Here's how the part is built. I have some questions about the finished solid (model axes, mm). A direction names the side the tool comes from. Coordinates: 2 decimals unless noted, no trailing zeros. Order: outer loops, then holes, each group sorted by start corner. A loop starts at its lowest first (then second) coordinate and runs counter-clockwise, first axis right, second up. Notation, with made-up numbers: (5, 8.25) - (31, 8.25) arc R9 ccw to (31, 18.25) - close; hole circle Ø6 at (48.5, 5). An arc over 180 degrees is marked (long way). Answer as CSV lines item,"result". Start each with the question number.
Item 1: Imagine slicing it at D-D on x = -51. List the corners of the cut face in (y, z) for me.
Item 2: We'd pull the mould along X, two halves only. Please class faces 6 (the face through (-71, 27, 0)), 7 (the face through (-101.483, 11.32, 3.131)), 8 (the face through (-46.732, 27, 3)): pulls with the +X half, pulls with the -X half, needs draft (parallel to the pull), parting line crosses it, or undercut.
Item 3: Imagine slicing it at A-A on x = -80.5. List the corners of the cut face in (y, z) for me, and give its area (3 significant figures).
Item 4: I need wall thicknesses on line 1 (X direction, y = 28, z = 6); line 2 (Y direction, x = -83, z = 2.25); line 3 (Y direction, x = -57, z = 6). Which ranges of each line are inside material? Lowest first, please.
Item 5: On a 3-axis mill with a long thin cutter (end or side, diameter ignored), from which of +Z, -Z, +X, -X, +Y, -Y can I reach the whole of each face in a straight line? I mean faces 1 (the face through (-70, 54.972, 3)), 2 (the face through (-75, -10, 3)), 3 (the face through (-60, -10, 3)), 4 (the face through (-68, 0, 3)), 5 (the face through (-71, 27, 6.35)). Say none if no direction works.
Item 6: I'm going to push a flat-ended pin straight in: pin 1 (4.5 mm diameter, centred on x = -67.06, y = 11.24, fed in from +Z). Where does the tip first touch, or does it pass through?
Item 7: Imagine slicing it at C-C on z = 2. Count the separate pieces of the cut face and the enclosed holes in it, and give its area (3 significant figures).
Item 8: Imagine slicing it at B-B on y = 50.5. List the corners of the cut face in (x, z) for me.
from build123d import *

# Parameters (mm, degrees)
SKETCH1_R           = 11
SKETCH1_R_2         = 1.89865
SKETCH1_R_3         = 1.9939
BOSS_EXTRUDE1_DEPTH = 6.35
FILLET1_R           = 10
SKETCH2_W           = 15
SKETCH2_H           = 19.05
BOSS_EXTRUDE2_DEPTH = 6.35
CHAMFER1_SIZE       = 1
SKETCH3_R           = 1
CUT_EXTRUDE1_DEPTH  = 159.045298363
SKETCH4_W           = 7.99338
SKETCH4_H           = 3.22072
CUT_EXTRUDE2_DEPTH  = 159.045298363
FILLET3_R           = 1
CUT_EXTRUDE3_DEPTH  = 159.045298363
FILLET4_R           = 10
SKETCH9_R           = 1
CUT_EXTRUDE4_DEPTH  = 124.871065449
FILLET5_R           = 1


with BuildPart() as part:
    # Sketch1 → Boss-Extrude1 (new body)
    with BuildSketch(Plane.XY):
        with BuildLine():
            Line((-40.498784978, 0), (0, 0))
            Line((0, 0), (0, 75))
            ThreePointArc((0, 75), (-37.5, 112.5), (-75, 75))
            Line((-75, 75), (-75, 55))
            Line((-75, 55), (-83.323029145, 55))
            ThreePointArc((-83.323029145, 55), (-110.823029145, 27.5), (-83.323029145, 0))
            Line((-83.323029145, 0), (-40.498784978, 0))
        make_face()
        with Locations((-83.323029145, 27.5)):
            Circle(SKETCH1_R, mode=Mode.SUBTRACT)
        with Locations((-67.059573177, 11.236544033)):
            Circle(SKETCH1_R_2, mode=Mode.SUBTRACT)
        with Locations((-83.323029145, 50.5)):
            Circle(SKETCH1_R_3, mode=Mode.SUBTRACT)
        with Locations((-99.586485112, 11.236544033)):
            Circle(SKETCH1_R_2, mode=Mode.SUBTRACT)
        with Locations((-60.323029145, 27.5)):
            Circle(SKETCH1_R_3, mode=Mode.SUBTRACT)
        with Locations((-99.586485112, 43.763455967)):
            Circle(SKETCH1_R_2, mode=Mode.SUBTRACT)
        with Locations((-83.323029145, 4.5)):
            Circle(SKETCH1_R_3, mode=Mode.SUBTRACT)
        with Locations((-106.323029145, 27.5)):
            Circle(SKETCH1_R_3, mode=Mode.SUBTRACT)
    extrude(amount=BOSS_EXTRUDE1_DEPTH)

    # Fillet1
    fillet1_edges = [part.edges().sort_by_distance(p)[0] for p in [
        (-75, 55, 3.175),
    ]]
    fillet(fillet1_edges, radius=FILLET1_R)

    # Sketch2 → Boss-Extrude2 (add)
    with BuildSketch(Plane(origin=(0, 0, 0), x_dir=(-1, 0, 0), z_dir=(0, 0, -1))):
        with Locations((7.5, -9.525)):
            Rectangle(SKETCH2_W, SKETCH2_H)
        with Locations((37.5, -9.525)):
            Rectangle(SKETCH2_W, SKETCH2_H)
        with Locations((67.5, -9.525)):
            Rectangle(SKETCH2_W, SKETCH2_H)
    extrude(amount=-BOSS_EXTRUDE2_DEPTH)

    # Chamfer1
    chamfer1_edges = [part.edges().sort_by_distance(p)[0] for p in [
        (0, -19.05, 3.175),
        (-15, -19.05, 3.175),
        (-30, -19.05, 3.175),
        (-45, -19.05, 3.175),
        (-60, -19.05, 3.175),
        (-75, -19.05, 3.175),
    ]]
    chamfer(chamfer1_edges, length=CHAMFER1_SIZE)

    # Sketch3 → Cut-Extrude1 (cut, through all)
    with BuildSketch(Plane.XY.offset(6.35)):
        with Locations((-75, 0)):
            Circle(SKETCH3_R)
        with Locations((-60, 0)):
            Circle(SKETCH3_R)
        with Locations((-45, 0)):
            Circle(SKETCH3_R)
        with Locations((-30, 0)):
            Circle(SKETCH3_R)
        with Locations((-15, 0)):
            Circle(SKETCH3_R)
    extrude(amount=-CUT_EXTRUDE1_DEPTH, mode=Mode.SUBTRACT)

    # Sketch4 → Cut-Extrude2 (cut, through all)
    with BuildSketch(Plane.XY.offset(6.35)):
        with Locations((-67.5, 1.61036)):
            Rectangle(SKETCH4_W, SKETCH4_H)
    extrude(amount=-CUT_EXTRUDE2_DEPTH, mode=Mode.SUBTRACT)

    # Fillet3
    fillet3_edges = [part.edges().sort_by_distance(p)[0] for p in [
        (-75, -1, 3.175),
        (-76, 0, 3.175),
        (-60, -1, 3.175),
        (-59, 0, 3.175),
        (-45, -1, 3.175),
        (-46, 0, 3.175),
        (-30, -1, 3.175),
        (-29, 0, 3.175),
        (-15, -1, 3.175),
        (-16, 0, 3.175),
    ]]
    fillet(fillet3_edges, radius=FILLET3_R)

    # Sketch5 → Cut-Extrude3 (cut, through all)
    with BuildSketch(Plane(origin=(0, 0, 0), x_dir=(-1, 0, 0), z_dir=(0, 0, -1))):
        Polygon((46.732050808, 0), (46.732050808, 54.972488867), (84.552807772, 54.972488867), (84.552807772, 112.5), (0, 112.5), (0, -19.05), (46.732050808, -19.05), align=None)
    extrude(amount=-CUT_EXTRUDE3_DEPTH, mode=Mode.SUBTRACT)

    # Fillet4
    fillet4_edges = [part.edges().sort_by_distance(p)[0] for p in [
        (-46.732050808, 0, 3.175),
        (-46.732050808, 54.972488867, 3.175),
    ]]
    fillet(fillet4_edges, radius=FILLET4_R)

    # Sketch9 → Cut-Extrude4 (cut, through all)
    with BuildSketch(Plane.XY.offset(6.35)):
        with Locations((-71.49669, 3.22072)):
            Circle(SKETCH9_R)
        with Locations((-63.50331, 3.22072)):
            Circle(SKETCH9_R)
        with Locations((-63.50331, 0)):
            Circle(SKETCH9_R)
        with Locations((-71.49669, 0)):
            Circle(SKETCH9_R)
    extrude(amount=-CUT_EXTRUDE4_DEPTH, mode=Mode.SUBTRACT)

    # Fillet5
    # the kernel refuses this fillet: 1 mm, written as the material it takes off along each edge
    with BuildSketch(Plane(origin=(-64.50331, 3.22072, -1.830127019), x_dir=(0.2588190451025049, 0.9659258262890725, 0), z_dir=(0, 0, 1)), Plane(origin=(-63.50331, 1, -1.830127019), x_dir=(0.9659258262890688, -0.25881904510251885, 0), z_dir=(0, 0, 1)), Plane(origin=(-71.49669, 2.22072, -1.830127019), x_dir=(-0.9659258262890682, 0.25881904510252124, 0), z_dir=(0, 0, 1))) as fillet5_piece_1:
        with BuildLine():
            CenterArc((0.776457135, 0.965925826), FILLET5_R, 195, 60)
            Line((-0.189468691, 0.707106781), (0, 0))
            ThreePointArc((0, 0), (0.258819045, 0.034074174), (0.51763809, 0))
        make_face()
    extrude(amount=10.010254038, mode=Mode.SUBTRACT)
    with BuildSketch(Plane(origin=(-63.50331, 2.22072, -1.830127019), x_dir=(0, -1, 0), z_dir=(0, 0, 1)), Plane(origin=(-71.49669, 1, -1.830127019), x_dir=(0, 1, 0), z_dir=(0, 0, 1))) as fillet5_piece_2:
        with BuildLine():
            CenterArc((0.732050808, 1), FILLET5_R, 210, 60)
            ThreePointArc((-0.133974596, 0.5), (-0.034074174, 0.258819045), (0, 0))
            Line((0, 0), (0.732050808, 0))
        make_face()
    extrude(amount=10.010254038, mode=Mode.SUBTRACT)
    with BuildSketch(Plane(origin=(-64.50331, 0, -1.830127019), x_dir=(0.2588190451025049, -0.9659258262890725, 0), z_dir=(0, 0, 1)), Plane(origin=(-70.49669, 0, 8.180127019), x_dir=(-0.25881904510253045, -0.9659258262890658, 0), z_dir=(0, 0, -1))) as fillet5_piece_3:
        with BuildLine():
            CenterArc((0.776457135, -0.965925826), FILLET5_R, 105, 60)
            Line((-0.189468691, -0.707106781), (0, 0))
            ThreePointArc((0, 0), (0.258819045, -0.034074174), (0.51763809, 0))
        make_face()
    extrude(amount=10.010254038, mode=Mode.SUBTRACT)
    with BuildSketch(Plane(origin=(-70.49669, 3.22072, 8.180127019), x_dir=(1, 0, 0), z_dir=(0, 0, -1))) as fillet5_piece_4:
        with BuildLine():
            CenterArc((0.732050808, -1), FILLET5_R, 90, 60)
            ThreePointArc((-0.133974596, -0.5), (-0.034074174, -0.258819045), (0, 0))
            Line((0, 0), (0.732050808, 0))
        make_face()
    extrude(amount=10.010254038, mode=Mode.SUBTRACT)


solid = part.part
Responses:
1,outline,"(1.81, 0) - (53.17, 0) - (53.17, 6.35) - (1.81, 6.35) - close"
2,face 6,"needs draft"
2,face 7,"undercut"
2,face 8,"pulls with the +X half"
3,outline,"(0, 0) - (16.87, 0) - (16.87, 6.35) - (0, 6.35) - close; (38.13, 0) - (54.97, 0) - (54.97, 6.35) - (38.13, 6.35) - close"
3,area,"214 mm^2"
4,line 1,"x = -110.82 to -108.25, -104.39 to -94.31, -72.33 to -62.25, -58.39 to -46.73"
4,line 2,"y = 0 to 2.53, 6.47 to 16.5, 38.5 to 48.53, 52.47 to 54.97"
4,line 3,"y = 0 to 54.97"
5,face 1,"+Z, -Z, +X, -X, +Y"
5,face 2,"+Z, -Z, -X, -Y"
5,face 3,"+Z, -Z, +X, -Y"
5,face 4,"+Z, -Z"
5,face 5,"+Z, +X, -X, +Y, -Y"
6,pin 1,"stops at z = 6.35"
7,separate pieces,"1"
7,enclosed holes,"9"
7,area,"2,940 mm^2"
8,outline,"(-98.4, 0) - (-85.32, 0) - (-85.32, 6.35) - (-98.4, 6.35) - close; (-81.33, 0) - (-48.4, 0) - (-48.4, 6.35) - (-81.33, 6.35) - close"
